Can you work these out from the drawing? Everything is in mm from the part's minimum corner. A direction names the side the tool comes from. Round coordinates to 2 decimals unless told otherwise and drop trailing zeros. Loops run counter-clockwise (first coordinate to the right, second up) from the corner with the lowest first, then second, coordinate; pieces in that order, holes last. Notation, with made-up numbers: (20.25, 86.25) - (42.25, 86.25) arc R20 ccw to (42.25, 98.25) - close; hole circle Ø4 at (8, -25.5). An arc over 180 degrees is marked (long way). Answer as a JSON object with one key per item and string values. Group by question number.
1) If I drill on line 1 along Z through (x, y) = (10, 89); line 2 along X through (y, z) = (31, 45), over which ranges is the centre line in solid material (lowest first)? Write a range as [from, to].
2) I want a section at B-B, the plane x = 35. Please give me the cut outline in (y, z).
3) I want a section at A-A, the plane y = 49.5. Please give me the cut outline in (x, z), then the cut area to 3 significant figures.
4) Will these pins go through, and if not, where does the flat tip stop? P1, Ø1, axis at x = 14, y = 63.5, coming from the +Z side; P2, Ø15, axis at y = 62.5, z = 61, coming from the -X side.
5) I want a section at C-C, the plane z = 36.5. Please give me the cut outline in (x, y).
6) Which directions (+Z, -Z, +X, -X, +Y, -Y) give clear straight access to the entire face, cutting with the end or side of a thin tool? Please do the marked faces 1 and 2.
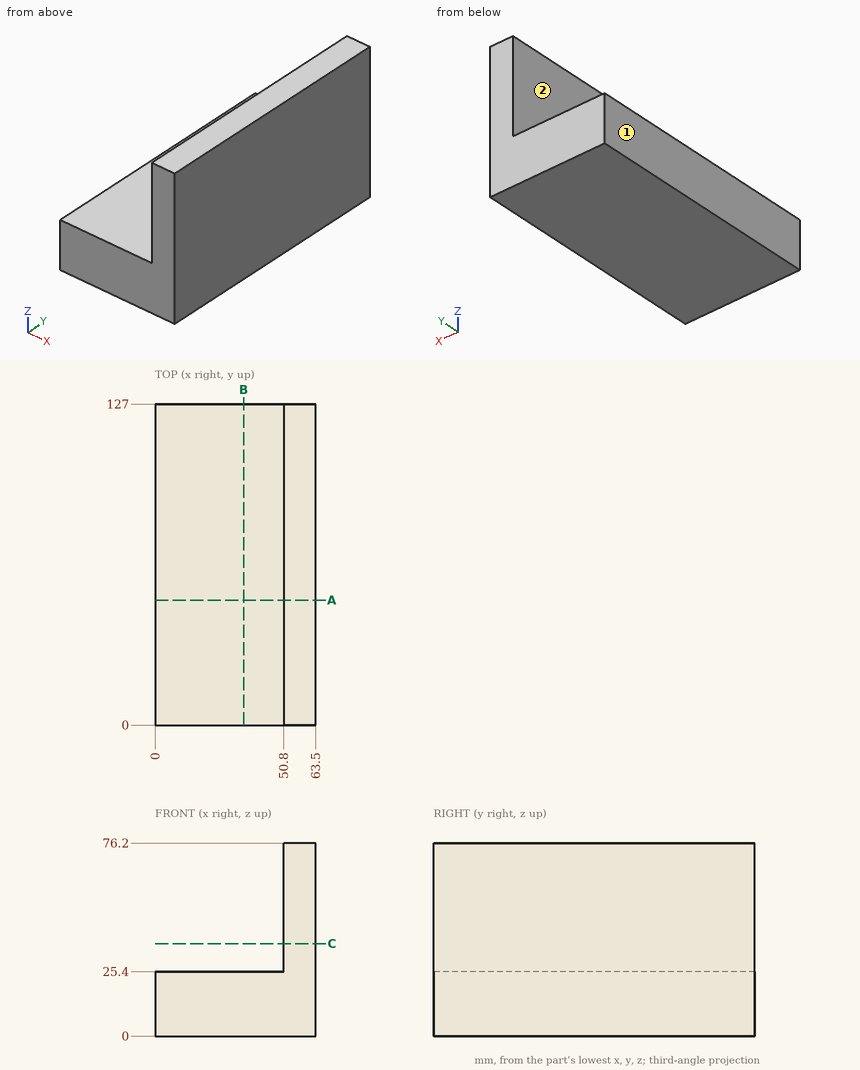
Outcome:
{
 "1": {"line 1": "[0, 25.4]", "line 2": "[50.8, 63.5]"},
 "2": {"outline": "(0, 0) - (127, 0) - (127, 25.4) - (0, 25.4) - close"},
 "3": {"outline": "(0, 0) - (63.5, 0) - (63.5, 76.2) - (50.8, 76.2) - (50.8, 25.4) - (0, 25.4) - close", "area": "2,260 mm^2"},
 "4": {"P1": "z = 25.4", "P2": "x = 50.8"},
 "5": {"outline": "(50.8, 0) - (63.5, 0) - (63.5, 127) - (50.8, 127) - close"},
 "6": {"face 1": "+Z, -Z, -X, +Y, -Y", "face 2": "+Z, -X, +Y, -Y"}
}
